```python
from build123d import *

# Parameters (mm, degrees)
CORPO_DEPTH                     = 15
REBAIXO_PARAFUSO_M4_D           = 4.5
REBAIXO_PARAFUSO_M4_DEPTH       = 30
REBAIXO_PARAFUSO_M4_CBORE_D     = 8
REBAIXO_PARAFUSO_M4_CBORE_DEPTH = 9
REBAIXO_PARAFUSO_M4_TIP         = 1.351936393


with BuildPart() as part:
    # Sketch1 → Corpo (new body)
    with BuildSketch(Plane.XY):
        with BuildLine():
            Line((16.252058195, 8.088672021), (23.764502557, 12.488672021))
            ThreePointArc((23.764502557, 12.488672021), (26.263743802, 12.734356122), (28.074119126, 10.993922652))
            ThreePointArc((28.074119126, 10.993922652), (30.15, 0), (28.074119126, -10.993922652))
            ThreePointArc((28.074119126, -10.993922652), (26.263743802, -12.734356122), (23.764502557, -12.488672021))
            Line((23.764502557, -12.488672021), (16.252058195, -8.088672021))
            ThreePointArc((16.252058195, -8.088672021), (14.971668435, -6.585929552), (14.902386515, -4.612903226))
            ThreePointArc((14.902386515, -4.612903226), (15.6, 0), (14.902386515, 4.612903226))
            ThreePointArc((14.902386515, 4.612903226), (14.971668435, 6.585929552), (16.252058195, 8.088672021))
        make_face()
    extrude(amount=CORPO_DEPTH)

    # Rebaixo - Parafuso M4
    with Locations(Plane.XY.offset(15)):
        with Locations((21.1, 0)):
            CounterBoreHole(REBAIXO_PARAFUSO_M4_D / 2, REBAIXO_PARAFUSO_M4_CBORE_D / 2, REBAIXO_PARAFUSO_M4_CBORE_DEPTH, depth=REBAIXO_PARAFUSO_M4_DEPTH)
            with Locations((0, 0, -(REBAIXO_PARAFUSO_M4_DEPTH + REBAIXO_PARAFUSO_M4_TIP / 2))):  # 118° drill point
                Cone(0, REBAIXO_PARAFUSO_M4_D / 2, REBAIXO_PARAFUSO_M4_TIP, mode=Mode.SUBTRACT)


solid = part.part
```
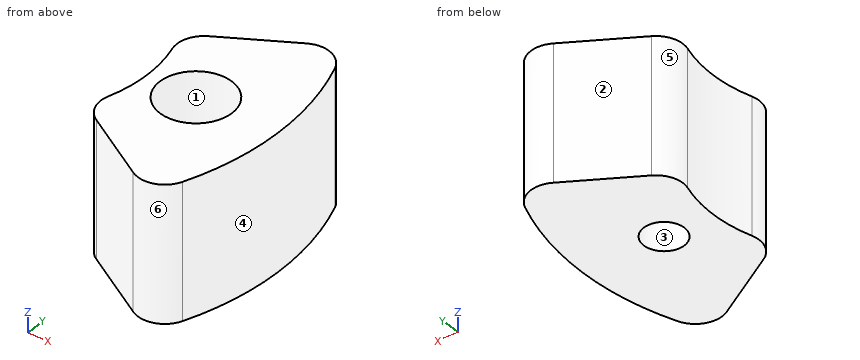
Geometry: final body of the model. Coordinates: model frame, mm. Face numbers are marked on the shaded views. A direction names the side the tool comes from. Round coordinates to 2 decimals unless told otherwise and drop trailing zeros. Loops run counter-clockwise (first coordinate to the right, second up) from the corner with the lowest first, then second, coordinate; pieces in that order, holes last.
Item 1: Section A-A, the plane z = 2. Output: boundary loops of the cut face in (x, y).
Checked values:
outline: (14.9, -4.61) arc R3 ccw to (16.25, -8.09) - (23.76, -12.49) arc R3 ccw to (28.07, -10.99) arc R30.15 ccw to (28.07, 10.99) arc R3 ccw to (23.76, 12.49) - (16.25, 8.09) arc R3 ccw to (14.9, 4.61) arc R15.6 cw to start; hole circle Ø4.5 at (21.1, 0)
Item 2: Section C-C, the plane x = 21. Output: boundary loops of the cut face in (y, z).
Checked values:
outline: (-10.87, 0) - (-2.25, 0) - (-2.25, 6) - (-4, 6) - (-4, 15) - (-10.87, 15) - close; (2.25, 0) - (10.87, 0) - (10.87, 15) - (4, 15) - (4, 6) - (2.25, 6) - close
Item 3: Line query: L1, parallel to Y at x = 21.1, z = 11.5; L2, parallel to Y at x = 20.25, z = 1.5; L3, parallel to X at y = 1.75, z = 5. Output: solid intervals per line, ascending.
Checked values:
L1: y = -10.93 to -4, 4 to 10.93
L2: y = -10.43 to -2.08, 2.08 to 10.43
L3: x = 15.5 to 19.69, 22.51 to 30.1
Item 4: Reachability of the marked faces 1 and 2 from +Z, -Z, +X, -X, +Y, -Y: full face, straight path, thin tool, end or side. Return the list, or none.
Checked values:
face 1: +Z
face 2: +Z, -Z, -X, +Y
Item 5: Section B-B, the plane y = 0. Output: boundary loops of the cut face in (x, z), plus the area to 3 significant figures.
Checked values:
outline: (15.6, 0) - (18.85, 0) - (18.85, 6) - (17.1, 6) - (17.1, 15) - (15.6, 15) - close; (23.35, 0) - (30.15, 0) - (30.15, 15) - (25.1, 15) - (25.1, 6) - (23.35, 6) - close
area: 119 mm2
Item 6: Mould query, pull axis Y, two halves, no side actions, for the marked faces 3, 4, 5 and 6. Classes: released by +Y, released by -Y, zero draft, split by the parting line, or undercut.
Checked values:
face 3: undercut
face 4: split by the parting line
face 5: undercut
face 6: released by -Y
Item 7: Section D-D, the plane z = 12. Output: boundary loops of the cut face in (x, y), plus the area to 3 significant figures.
Checked values:
outline: (14.9, -4.61) arc R3 ccw to (16.25, -8.09) - (23.76, -12.49) arc R3 ccw to (28.07, -10.99) arc R30.15 ccw to (28.07, 10.99) arc R3 ccw to (23.76, 12.49) - (16.25, 8.09) arc R3 ccw to (14.9, 4.61) arc R15.6 cw to start; hole circle Ø8 at (21.1, 0)
area: 259 mm2
Item 8: Contact query for flat-ended pins moving along their axis: P1, Ø1, axis at y = -4.5, z = 3, coming from the -X side; P2, Ø4, axis at x = 20.5, z = 4.5, coming from the +Y side; P3, Ø1, axis at x = 27.5, z = 12.5, coming from the -Y side. Output: stop coordinate, or through.
Checked values:
P1: stops at x = 14.81
P2: stops at y = 11.75
P3: stops at y = -12.36
